```python
from build123d import *

# Parameters (mm, degrees)
SKETCH_1_R          = 3
EXTRUDE_1_DEPTH     = 8
EXTRUDE_1_2_DEPTH   = 8
SKETCH_1_3_R        = 17
SKETCH_1_3_R_2      = 8
EXTRUDE_2_DEPTH     = 20
EXTRUDE_3_REACH     = 39
SKETCH_2_W          = 20
SKETCH_2_H          = 20
SKETCH_3_W          = 20
SKETCH_3_H          = 2
CUT_EXTRUDE_1_DEPTH = 20
SKETCH_4_R          = 2.5
CUT_EXTRUDE_2_DEPTH = 41


with BuildPart() as part:
    # Sketch 1 → Extrude 1 (new body)
    with BuildSketch(Plane(origin=(0, 0, 0), x_dir=(0, 0, -1), z_dir=(1, 0, 0))):
        with BuildLine():
            Line((-7.18451045, 15.40723238), (-30, 4.768194878))
            Line((-30, 4.768194878), (-30, -4.768194878))
            Line((-30, -4.768194878), (-7.18451045, -15.40723238))
            ThreePointArc((-7.18451045, -15.40723238), (-17, 0), (-7.18451045, 15.40723238))
        make_face()
        with Locations((-24, 0)):
            Circle(SKETCH_1_R, mode=Mode.SUBTRACT)
    extrude(amount=EXTRUDE_1_DEPTH)



with BuildPart() as body_2:
    # Sketch 1 → Extrude 1 2 (new body)
    with BuildSketch(Plane(origin=(0, 0, 0), x_dir=(0, 0, -1), z_dir=(1, 0, 0))):
        with BuildLine():
            Line((30, 4.768194878), (7.18451045, 15.40723238))
            ThreePointArc((7.18451045, 15.40723238), (14.337654579, 9.134093342), (17, 0))
            ThreePointArc((17, 0), (14.337654579, -9.134093342), (7.18451045, -15.40723238))
            Line((7.18451045, -15.40723238), (30, -4.768194878))
            Line((30, -4.768194878), (30, 4.768194878))
        make_face()
        with Locations((24, 0)):
            Circle(SKETCH_1_R, mode=Mode.SUBTRACT)
    extrude(amount=EXTRUDE_1_2_DEPTH)


with BuildPart() as part_1:
    add(part.part)

    add(body_2.part)  # Extrude 2 merges body 2
    # Sketch 1_3 → Extrude 2 (add)
    with BuildSketch(Plane(origin=(0, 0, 0), x_dir=(0, 0, -1), z_dir=(1, 0, 0))):
        Circle(SKETCH_1_3_R)
        Circle(SKETCH_1_3_R_2, mode=Mode.SUBTRACT)
    extrude(amount=EXTRUDE_2_DEPTH)

    # Sketch 2 → Extrude 3 (add, up to next)
    with BuildSketch(Plane(origin=(0, 20, 0), x_dir=(1, 0, 0), z_dir=(0, 1, 0)), mode=Mode.PRIVATE) as extrude_3_sk1:
        with Locations((10, 0)):
            Rectangle(SKETCH_2_W, SKETCH_2_H)
    extrude_3_tool1 = extrude(extrude_3_sk1.sketch, amount=-EXTRUDE_3_REACH, mode=Mode.PRIVATE) - part_1.part
    add(extrude_3_tool1.solids().sort_by_distance((10, 20, 0))[0])

    # Sketch 3 → Cut-Extrude 1 (cut)
    with BuildSketch(Plane(origin=(0, 20, 0), x_dir=(1, 0, 0), z_dir=(0, 1, 0))):
        with Locations((10, 0)):
            Rectangle(SKETCH_3_W, SKETCH_3_H)
    extrude(amount=-CUT_EXTRUDE_1_DEPTH, mode=Mode.SUBTRACT)

    # Sketch 4 → Cut-Extrude 2 (cut, through all)
    with BuildSketch(Plane.XY.offset(10)):
        with Locations((10, 17)):
            Circle(SKETCH_4_R)
    extrude(amount=-CUT_EXTRUDE_2_DEPTH, mode=Mode.SUBTRACT)


solid = part_1.part
```
Verification items for the finished model (mm, model axes). A direction names the side the tool comes from. Round coordinates to 2 decimals unless told otherwise and drop trailing zeros. Order: outer loops, then holes, each group sorted by start corner. A loop starts at its lowest first (then second) coordinate and runs counter-clockwise, first axis right, second up.
1) Cross-section at B-B, the plane y = 0. Record the cut outline in (x, z).
Geometry says:
outline: (0, -30) - (8, -30) - (8, -27) - (0, -27) - close; (0, -21) - (8, -21) - (8, -17) - (20, -17) - (20, -8) - (0, -8) - close; (0, 8) - (20, 8) - (20, 17) - (8, 17) - (8, 21) - (0, 21) - close; (0, 27) - (8, 27) - (8, 30) - (0, 30) - close
2) Cross-section at D-D, the plane z = 5.5. Record the cut outline in (x, y), plus the area to 3 significant figures.
Geometry says:
outline: (0, -16.09) - (20, -16.09) - (20, -5.81) - (0, -5.81) - close; (0, 5.81) - (20, 5.81) - (20, 20) - (0, 20) - close; hole circle Ø5 at (10, 17)
area: 470 mm2
3) Tool access check on faces 5 (the cylindrical face through (14.3, -16.99, 0.6)), 6 (the flat face through (10, 14, -1)), 7 (the flat face through (3.944, -10.162, -18.433)). Record the directions out of +Z, -Z, +X, -X, +Y, -Y that give a thin tool (end or side, any length) a straight path to the whole face; none if there is none.
Geometry says:
face 5: +X
face 6: +X, -X, +Y
face 7: -Z, +X, -X, -Y
4) Material ranges on line 1 (Y direction, x = 10, z = 5) (3 decimals); line 2 (Y direction, x = 8.5, z = -6); line 3 (Z direction, x = 14.75, y = 0), recorded low to high.
Geometry says:
line 1: y = -16.248 to -6.245, 6.245 to 14.5, 19.5 to 20
line 2: y = -15.91 to -5.29, 5.29 to 15, 19 to 20
line 3: z = -17 to -8, 8 to 17
5) Draft check along Y on faces 1 (the cylindrical face through (10, -8, 0)), 2 (the flat face through (3.944, -10.013, 18.752)), 3 (the flat face through (4, 0, -30)), 4 (the flat face through (3.944, 9.497, 19.86)). Enter one of: +Y half, -Y half, draft (parallel to the pull), parting line (faces both ways), or undercut.
Geometry says:
face 1: undercut
face 2: -Y half
face 3: draft
face 4: +Y half
6) Depth check by flat-ended pin: pin 1 (7 mm diameter, centred on x = 13.5, y = 16.5, fed in from -Z); pin 2 (12 mm diameter, centred on x = 14.5, y = -4, fed in from +Z); pin 3 (2 mm diameter, centred on x = 7.5, y = 8, fed in from -Z); pin 4 (4 mm diameter, centred on x = 10, y = 17, fed in from -Z). Enter the tip coordinate at first touch or a pass-through.
Geometry says:
pin 1: stops at z = -10.95
pin 2: stops at z = 17
pin 3: stops at z = -25.21
pin 4: passes through
7) Cross-section at C-C, the plane x = 1.5. Record the cut outline in (y, z).
Geometry says:
outline: (-15.41, -7.18) - (-4.77, -30) - (4.77, -30) - (14.09, -10) - (20, -10) - (20, -1) - (7.94, -1) arc R8 cw (long way) to (7.94, 1) - (20, 1) - (20, 10) - (14.09, 10) - (4.77, 30) - (-4.77, 30) - (-15.41, 7.18) arc R17 ccw to start; hole circle Ø6 at (0, -24); hole circle Ø6 at (0, 24)
8) Cross-section at A-A, the plane x = 10. Record the cut outline in (y, z).
Geometry says:
outline: (7.94, -1) arc R8 cw (long way) to (7.94, 1) - (14.5, 1) - (14.5, 10) - (13.75, 10) arc R17 ccw (long way) to (13.75, -10) - (14.5, -10) - (14.5, -1) - close; (19.5, -10) - (20, -10) - (20, -1) - (19.5, -1) - close; (19.5, 1) - (20, 1) - (20, 10) - (19.5, 10) - close
